The model under review builds one solid part; all positions refer to its coordinate system, in mm. A direction names the side the tool comes from. Coordinates: 2 decimals unless noted, no trailing zeros. Order: outer loops, then holes, each group sorted by start corner. A loop starts at its lowest first (then second) coordinate and runs counter-clockwise, first axis right, second up. Notation, with made-up numbers: M -18.5,36 L 14.5,36 A22 ccw 14.5,64 Z; hole C 81.5,44.5 d6. An arc over 180 degrees is marked long. One line per item, written item: value.
```python
from build123d import *

# Parameters (mm, degrees)
BOSS_EXTRUDE1_DEPTH     = 40
FILLET1_R               = 220
FILLET2_R               = 30
CUT_EXTRUDE1_DEPTH      = 1391.71923838
CUT_EXTRUDE1_DEPTH_BACK = 1391.71923838
FILLET3_R               = 10


with BuildPart() as part:
    # Sketch1 → Boss-Extrude1 (new body)
    with BuildSketch(Plane(origin=(0, 0, 0), x_dir=(1, 0, 0), z_dir=(0, 1, 0))):
        Polygon((850, 1100), (-850, 1100), (-850, 0), (-400, 0), (-400, 450), (400, 450), (400, 0), (850, 0), align=None)
    extrude(amount=BOSS_EXTRUDE1_DEPTH)

    # Fillet1
    fillet1_edges = [part.edges().sort_by_distance(p)[0] for p in [
        (-400, 20, -450),
        (-400, 20, 0),
        (400, 20, 0),
        (400, 20, -450),
    ]]
    fillet(fillet1_edges, radius=FILLET1_R)

    # Fillet2
    fillet2_edges = [part.edges().sort_by_distance(p)[0] for p in [
        (-850, 20, 0),
        (-850, 20, -1100),
        (850, 20, -1100),
        (850, 20, 0),
    ]]
    fillet(fillet2_edges, radius=FILLET2_R)

    # Sketch2 → Cut-Extrude1 (cut, two sides: drawn at the far end of the back side and taken through both)
    with BuildSketch(Plane(origin=(0, 40, 0), x_dir=(1, 0, 0), z_dir=(0, 1, 0)).offset(-CUT_EXTRUDE1_DEPTH_BACK)):
        Polygon((-15, 3908.73185568), (-15, 1100), (-15, 1070), (-40, 1070), (-40, 1040), (40, 1040), (40, 1070), (15, 1070), (15, 1100), (15, 3908.73185568), (15, 9526.195567041), (-15, 9526.195567041), align=None)
    extrude(amount=CUT_EXTRUDE1_DEPTH + CUT_EXTRUDE1_DEPTH_BACK, mode=Mode.SUBTRACT)

    # Fillet3
    fillet3_edges = [part.edges().sort_by_distance(p)[0] for p in [
        (-15, 20, -1070),
        (-40, 20, -1070),
        (-40, 20, -1040),
        (40, 20, -1040),
        (40, 20, -1070),
        (15, 20, -1070),
        (15, 20, -1100),
        (-15, 20, -1100),
    ]]
    fillet(fillet3_edges, radius=FILLET3_R)


solid = part.part
```
(1) Tool access review of faces 4 (the flat face through (428, 20, -1100)), 5 (the cylindrical face through (-337.265, 20.28, -383.844)), 6 (the flat face through (0, 20, -1040)): name each direction out of +Z, -Z, +X, -X, +Y, -Y from which nothing blocks a thin tool from reaching the whole face with its end or side.
Geometry results:
face 4: -Z, +X, -X, +Y, -Y
face 5: +Z, +Y, -Y
face 6: +Y, -Y
(2) We need section C-C, the plane z = -189. State the section outline as (x, y) points.
Geometry results:
outline: M -850,0 L -402.2,0 L -402.2,40 L -850,40 Z; M 402.2,0 L 850,0 L 850,40 L 402.2,40 Z
(3) We need section D-D, the plane x = 260. State the section outline as (y, z) points.
Geometry results:
outline: M 0,-1100 L 40,-1100 L 40,-434.94 L 0,-434.94 Z
(4) Insertion check: pin 1 Ø2.5 at (x, y) = (27, 11.5) entering from +Z; pin 2 Ø8 at (y, z) = (16, -1084) entering from -X; pin 3 Ø3 at (y, z) = (16, -1084) entering from +X. Each pin has a flat end and moves straight along its axis. Give the tip position at first contact, or say it passes through.
Geometry results:
pin 1: stops at z = -450
pin 2: stops at x = -848.28
pin 3: stops at x = 847.27
(5) We need section B-B, the plane z = -328.5. State the section outline as (x, y) points, plus the area to 3 significant figures.
Geometry results:
outline: M -850,0 L -376.72,0 L -376.72,40 L -850,40 Z; M 376.72,0 L 850,0 L 850,40 L 376.72,40 Z
area: 37,900 mm2
(6) For L1, parallel to X at y = 22, z = -1048.5; L2, parallel to X at y = 34, z = -158; L3, parallel to Z at x = -12, y = 32, list the stretches that pass through material, from the lowest coordinate up.
Geometry results:
L1: x = -850 to -39.89, 39.89 to 850
L2: x = -850 to -408.92, 408.92 to 850
L3: z = -1040 to -450
(7) Mouldability with a two-part tool opening along X and no side actions: class faces 1 (the flat face through (-721, 20, 0)), 2 (the flat face through (-850, 20, -557)), 3 (the flat face through (-3, 20, -450)) as +X half, -X half, draft (parallel to the pull), parting line (faces both ways), or undercut.
Geometry results:
face 1: draft
face 2: -X half
face 3: undercut
